Check sheet for the drawn part. Datum: minimum x, y, z corner. Units: mm. Give positions to 0.01 mm unless a question says otherwise; leave off trailing zeros. Order: outer loops, then holes, each group sorted by start corner. A loop starts at its lowest first (then second) coordinate and runs counter-clockwise, first axis right, second up. Notation, with made-up numbers: (18, 41.25) -> (69, 41.25) arc R24 ccw to (69, 54.25) -> close; hole circle Ø4 at (3.5, 40). An arc over 180 degrees is marked (long way). One line per question, with ' | ' between items. Start each with the question number.
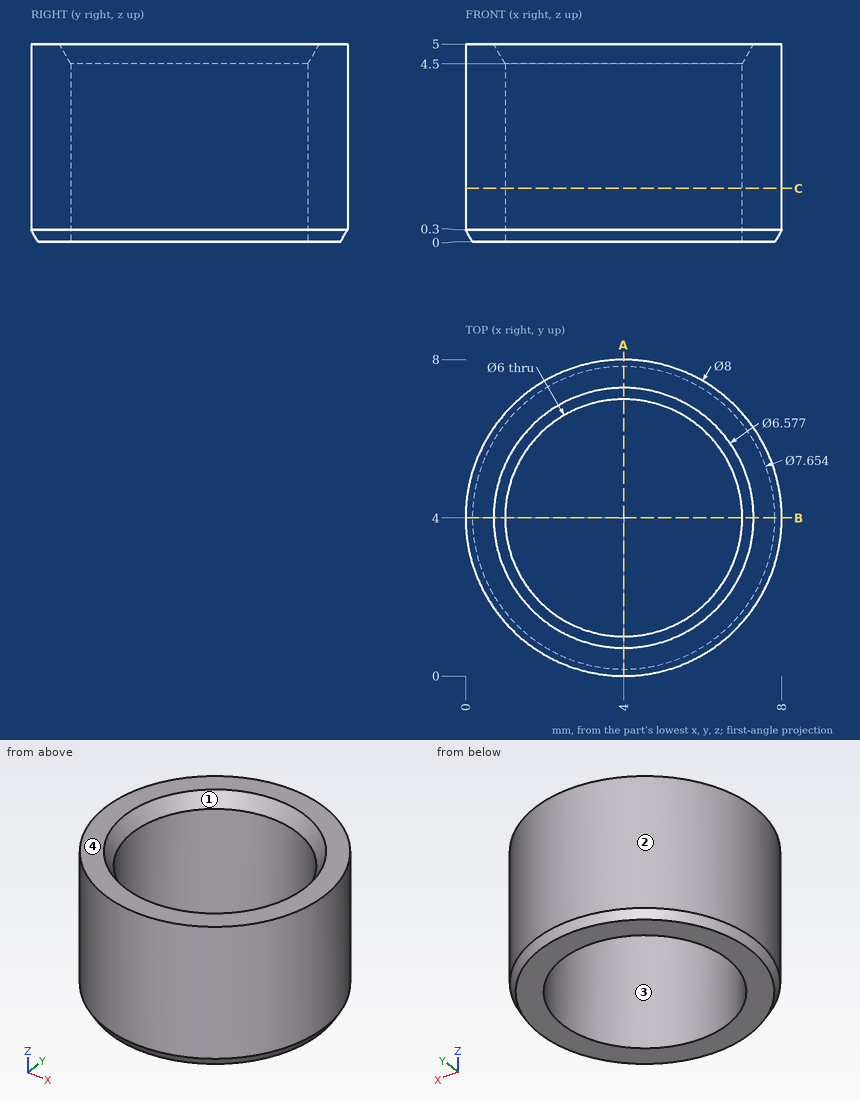
1. Mould release check, pull along X, two halves, no side actions. Record for the marked faces 1, 2, 3 and 4: +X half, -X half, draft (parallel to the pull), parting line (faces both ways), or undercut.
2. Cross-section at A-A on x = 4. Record the boundary of the cut face in (y, z).
3. Scan lines: probe 1 along Y at (x, z) = (4, 2.1); probe 2 along X at (y, z) = (6, 1.05) (1 decimal); probe 3 along X at (y, z) = (2.25, 4.1) (1 decimal). Record each from-to range of solid material in increasing order.
4. Cross-section at C-C on z = 1.35. Record the boundary of the cut face in (x, y), and give its area (3 significant figures).
Response values:
1) face 1: undercut | face 2: parting line | face 3: undercut | face 4: draft
2) outline: (0, 0.3) -> (0.17, 0) -> (1, 0) -> (1, 4.5) -> (0.71, 5) -> (0, 5) -> close; (7, 0) -> (7.83, 0) -> (8, 0.3) -> (8, 5) -> (7.29, 5) -> (7, 4.5) -> close
3) probe 1: y = 0 to 1, 7 to 8 | probe 2: x = 0.5 to 1.8, 6.2 to 7.5 | probe 3: x = 0.4 to 1.6, 6.4 to 7.6
4) outline: circle Ø8 at (4, 4); hole circle Ø6 at (4, 4) | area: 22.0 mm²
